```python
from build123d import *

# Parameters (mm, degrees)
SKETCH1_W           = 762
SKETCH1_H           = 762
BOSS_EXTRUDE1_DEPTH = 203.2
CUT_EXTRUDE1_DEPTH  = 101.6
SKETCH4_W           = 203.2
SKETCH4_H           = 508
CUT_EXTRUDE2_DEPTH  = 76.2
SKETCH6_R           = 12.7
CUT_EXTRUDE3_DEPTH  = 939.426022657
FILLET2_R           = 43.18
SKETCH10_R          = 50.8
BOSS_EXTRUDE2_DEPTH = 17.78
FILLET3_R           = 10.16
FILLET4_R           = 10.16


# Read off the part's stored shape, not the designer's step: Revolve2
with BuildPart() as part:
    # Sketch1 → Boss-Extrude1 (new body)
    with BuildSketch(Plane(origin=(0, 0, 0), x_dir=(1, 0, 0), z_dir=(0, 1, 0))):
        with Locations((254, 0)):
            Rectangle(SKETCH1_W, SKETCH1_H)
    extrude(amount=BOSS_EXTRUDE1_DEPTH)

    # Sketch3 → Cut-Extrude1 (cut)
    with BuildSketch(Plane.XY.offset(381)):
        Polygon((200.323484187, 101.6), (53.676515813, 101.6), (-19.646968374, -25.4), (53.676515813, -152.4), (200.323484187, -152.4), (273.646968374, -25.4), align=None)
    cut_extrude1 = extrude(amount=-CUT_EXTRUDE1_DEPTH, mode=Mode.SUBTRACT)

    # Mirror1: Cut-Extrude1 across plane
    add(cut_extrude1.mirror(Plane.XY), mode=Mode.SUBTRACT)

    # Sketch4 → Cut-Extrude2 (cut)
    with BuildSketch(Plane.XZ):
        with Locations((127, 0)):
            Rectangle(SKETCH4_W, SKETCH4_H)
    extrude(amount=-CUT_EXTRUDE2_DEPTH, mode=Mode.SUBTRACT)

    # Sketch6 → Cut-Extrude3 (cut, through all)
    with BuildSketch(Plane.XY.offset(279.4)):
        with Locations(Location((127, 20.32, 0), (0, 0, 180))):
            Circle(SKETCH6_R)
    extrude(amount=-CUT_EXTRUDE3_DEPTH, mode=Mode.SUBTRACT)

    # Fillet2
    fillet2_edges = [part.edges().sort_by_distance(p)[0] for p in [
        (-4.982271537, 0, 330.2),
        (258.982271537, 0, 330.2),
        (200.323484187, 101.6, 330.2),
        (53.676515813, 101.6, 330.2),
        (-4.982271537, 0, -330.2),
        (258.982271537, 0, -330.2),
        (53.676515813, 101.6, -330.2),
        (200.323484187, 101.6, -330.2),
    ]]
    fillet(fillet2_edges, radius=FILLET2_R)

    # Sketch10 → Boss-Extrude2 (add)
    with BuildSketch(Plane.XZ):
        with Locations(Location((558.8, 0, 0), (0, 0, 90))):
            Circle(SKETCH10_R)
    extrude(amount=BOSS_EXTRUDE2_DEPTH)

    # Sketch12 → Cut-Revolve3 (revolve, cut)
    with BuildSketch(Plane(origin=(0, -17.78, 0), x_dir=(-1, 0, 0), z_dir=(0, -1, 0))):
        with BuildLine():
            Line((-520.7, 0), (-596.9, 0))
            ThreePointArc((-596.9, 0), (-558.8, -38.1), (-520.7, 0))
        make_face()
    revolve(axis=Axis((520.7, -17.78, 0), (1, 0, 0)), mode=Mode.SUBTRACT)

    # Revolve2 outline → Revolve2 (revolve)
    with BuildSketch(Plane(origin=(558.8, 0, 0), x_dir=(1, 0, 0), z_dir=(0, 0, 1))):
        with BuildLine():
            ThreePointArc((38.1, -17.77999996), (36.04252118, -30.130978383), (30.092300919, -41.14800003))
            Line((30.092300919, -41.14800003), (31.071167059, -43.180000031))
            ThreePointArc((31.071167059, -43.180000031), (37.79897817, -31.263867149), (40.132, -17.77999996))
            Line((40.132, -17.77999996), (38.1, -17.77999996))
        make_face()
    revolve(axis=Axis((558.8, 0, 0), (0, 1, 0)))

    # Fillet3
    fillet3_edges = [part.edges().sort_by_distance(p)[0] for p in [
        (558.8, -17.78, -50.8),
    ]]
    fillet(fillet3_edges, radius=FILLET3_R)

    # Fillet4
    fillet4_edges = [part.edges().sort_by_distance(p)[0] for p in [
        (635, 0, 0),
    ]]
    fillet(fillet4_edges, radius=FILLET4_R)


solid = part.part
```
Here's how the part is built. I have some questions about the finished solid (model axes, mm). A direction names the side the tool comes from. Coordinates: 2 decimals unless noted, no trailing zeros. Write each loop counter-clockwise with the first axis right and the second up, starting at its lowest first coordinate (ties: lowest second). Pieces come first, ordered by that corner, then holes. Notation, with made-up numbers: (64, 64) -> (113, 64) arc R25 cw to (113, 83) -> close; hole circle Ø2 at (-6.75, 17.5). An arc over 180 degrees is marked (long way). Use a Markdown table: item, result. Add a question column.
(1) For faces 1 (the flat face through (128, 101.6, -331)), 2 (the flat face through (635, 105, 5)), 3 (the cylindrical face through (56.743, 95.656, 329.489)), which set-ups out of +Z, -Z, +X, -X, +Y, -Y let a thin tool reach every point of the face, with its end or its side?
(2) If we section it at C-C, the plane z = 300.5: Write out the boundary of the cut face in (x, y), and give its area (3 significant figures).
(3) If we section it at B-B, the plane y = 49: Write out the boundary of the cut face in (x, z).
(4) Please list where these lines run through material, in increasing order: line 1 (X direction, y = 47.5, z = -161); line 2 (X direction, y = 20.32, z = -266.5); line 3 (Y direction, x = 127, z = 262).
(5) We'd pull the mould along Z, two halves only. Please class faces 4 (the flat face through (125, 52, 279.4)), 5 (the flat face through (25.4, 38, -4)), 6 (the flat face through (125, 52, -279.4)), 7 (the flat face through (128, 101.6, 331)): +Z half, -Z half, draft (parallel to the pull), parting line (faces both ways), or undercut.
(6) If we section it at D-D, the plane x = 274.5: Write out the boundary of the cut face in (y, z).
(7) If we section it at A-A, the plane x = 127: Write out the boundary of the cut face in (y, z), and give its area (3 significant figures).
(8) I'm going to push flat-ended pins straight in: P1, Ø15, axis at x = 127, y = 20.32, coming from the -Z side; P2, Ø6, axis at x = 112, y = 76.5, coming from the +Z side; P3, Ø23, axis at x = 96, y = 29.5, coming from the -Z side; P4, Ø6, axis at x = 489, z = -284, coming from the -Y side. Where does each tip first touch, or does it pass through?
Outcome:
| question | item | result |
|---|---|---|
| 1 | face 1 | -Z, -Y |
| 1 | face 2 | +Z, -Z, +X, +Y, -Y |
| 1 | face 3 | +Z, -Y |
| 2 | outline | (-127, 0) -> (-29.91, 0) arc R43.18 ccw to (7.48, 21.59) -> (41.21, 80.01) arc R43.18 cw to (78.61, 101.6) -> (175.39, 101.6) arc R43.18 cw to (212.79, 80.01) -> (246.52, 21.59) arc R43.18 ccw to (283.91, 0) -> (624.84, 0) arc R10.16 ccw to (635, 10.16) -> (635, 203.2) -> (-127, 203.2) -> close |
| 2 | area | 134,000 mm^2 |
| 3 | outline | (-127, -381) -> (23.31, -381) -> (23.31, -279.4) -> (230.69, -279.4) -> (230.69, -381) -> (635, -381) -> (635, 381) -> (230.69, 381) -> (230.69, 279.4) -> (23.31, 279.4) -> (23.31, 381) -> (-127, 381) -> close; hole (25.4, -254) -> (228.6, -254) -> (228.6, 254) -> (25.4, 254) -> close |
| 4 | line 1 | x = -127 to 25.4, 228.6 to 635 |
| 4 | line 2 | x = -127 to 114.3, 139.7 to 635 |
| 4 | line 3 | y = 0 to 7.62, 33.02 to 203.2 |
| 5 | face 4 | +Z half |
| 5 | face 5 | undercut |
| 5 | face 6 | -Z half |
| 5 | face 7 | draft |
| 6 | outline | (0, -279.4) -> (1.04, -279.4) -> (1.04, -381) -> (203.2, -381) -> (203.2, 381) -> (1.04, 381) -> (1.04, 279.4) -> (0, 279.4) -> close |
| 7 | outline | (0, -279.4) -> (7.62, -279.4) -> (7.62, -254) -> (0, -254) -> close; (0, 254) -> (7.62, 254) -> (7.62, 279.4) -> (0, 279.4) -> close; (33.02, -279.4) -> (101.6, -279.4) -> (101.6, -381) -> (203.2, -381) -> (203.2, 381) -> (101.6, 381) -> (101.6, 279.4) -> (33.02, 279.4) -> (33.02, 254) -> (76.2, 254) -> (76.2, -254) -> (33.02, -254) -> close |
| 7 | area | 94,200 mm^2 |
| 8 | P1 | passes through |
| 8 | P2 | stops at z = 279.4 |
| 8 | P3 | stops at z = -279.4 |
| 8 | P4 | stops at y = 0 |
